Work out the finished part from the listing and answer in its coordinate system (mm). Face numbers are marked on the shaded views. Give positions to 0.01 mm unless a question says otherwise; leave off trailing zeros. Order: outer loops, then holes, each group sorted by start corner. A loop starts at its lowest first (then second) coordinate and runs counter-clockwise, first axis right, second up. Notation, with made-up numbers: (60, 75.25) -> (94, 75.25) arc R12 ccw to (94, 82.25) -> close; hole circle Ø2 at (21, 30). An arc over 180 degrees is marked (long way). Answer as CSV lines item,"result". Start each with the question number.
1. For a pull along X with two mould halves and no side action, classify the marked faces 1, 2 and 3 as released by +X, released by -X, zero draft, split by the parting line, or undercut.
2. A flat-ended cylindrical pin translates along its axis: pin 1 (2 mm diameter, centred on y = 13.5, z = 1.5, fed in from +X). Find the tip coordinate at first contact, or state that the pin passes through.
3. A cutting plane is placed at B-B (z = 2.5). State how many separate pieces and enclosed holes the cut face has, then the cut area to 3 significant figures.
4. A cutting plane is placed at A-A (x = -2). Give the vertices of the cut face in (y, z).
5. Find the intervals of material crossed by L1, parallel to X at y = -19, z = 4.5; L2, parallel to Y at x = -8, z = 2.2; L3, parallel to X at y = 24.5, z = 3.4, in increasing order.
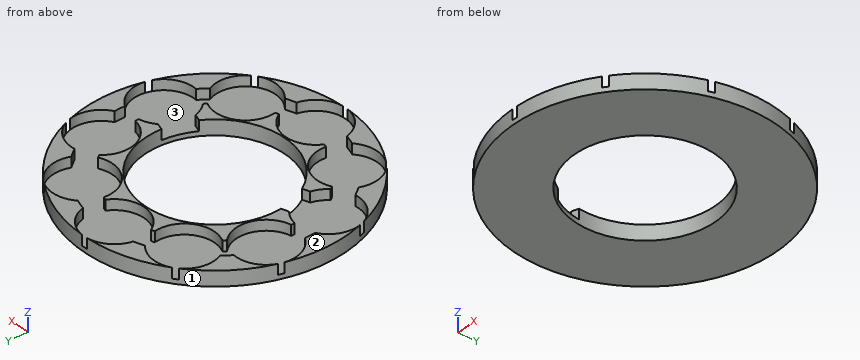
from build123d import *

# Parameters (mm, degrees)
SKETCH1_R                  = 42.14825
SKETCH1_R_2                = 22.5
BASIC_SHAPE_DEPTH          = 4.8
SKETCH2_R                  = 9.65
BATTERY_SLOT_DEPTH         = 3.3
BATTERY_SLOT_PATTERN_COUNT = 10
SKETCH3_R                  = 35.78
SKETCH3_R_2                = 29.28
BUS_SLOT_DEPTH             = 3.3
WIRE_SLIT_DEPTH            = 3.3


with BuildPart() as part:
    # Sketch1 → Basic Shape (new body)
    with BuildSketch(Plane.XY):
        Circle(SKETCH1_R)
        Circle(SKETCH1_R_2, mode=Mode.SUBTRACT)
    extrude(amount=BASIC_SHAPE_DEPTH)

    # Sketch2 → Battery Slot (cut)
    with BuildSketch(Plane.XY.offset(4.8)):
        with Locations((0, -32.53)):
            Circle(SKETCH2_R)
    battery_slot = extrude(amount=-BATTERY_SLOT_DEPTH, mode=Mode.SUBTRACT)

    # Battery Slot Pattern: Battery Slot ×10 about axis
    battery_slot_pattern_axis = Axis((0, 0, 0), (0, 0, 1))
    for i in range(1, BATTERY_SLOT_PATTERN_COUNT):
        add(battery_slot.rotate(battery_slot_pattern_axis, i * 360 / BATTERY_SLOT_PATTERN_COUNT), mode=Mode.SUBTRACT)

    # Sketch3 → Bus Slot (cut)
    with BuildSketch(Plane.XY.offset(4.8)):
        Circle(SKETCH3_R)
        Circle(SKETCH3_R_2, mode=Mode.SUBTRACT)
    extrude(amount=-BUS_SLOT_DEPTH, mode=Mode.SUBTRACT)

    # Sketch4 → Wire Slit (cut)
    with BuildSketch(Plane.XY.offset(4.8)):
        with BuildLine():
            Line((-24.633279562, -2.746526591), (-19.877996981, -1.201441619))
            Line((-19.877996981, -1.201441619), (-16.787827037, -10.712006782))
            Line((-16.787827037, -10.712006782), (-21.543109618, -12.257091754))
            ThreePointArc((-21.543109618, -12.257091754), (-21.760173093, -7.070308831), (-24.633279562, -2.746526591))
        make_face()
    wire_slit = extrude(amount=-WIRE_SLIT_DEPTH, mode=Mode.SUBTRACT)

    # Wire Slit Mirror: Wire Slit across plane
    add(wire_slit.mirror(Plane(origin=(0, 0, 0), x_dir=(0, 0, 1), z_dir=(1, 0, 0))), mode=Mode.SUBTRACT)


solid = part.part
Answer sheet:
1,face 1,"split by the parting line"
1,face 2,"zero draft"
1,face 3,"undercut"
2,pin 1,"stops at x = 40.25"
3,separate pieces,"12"
3,enclosed holes,"0"
3,area,"951 mm^2"
4,outline,"(-42.1, 0) -> (-22.41, 0) -> (-22.41, 4.8) -> (-23.09, 4.8) -> (-23.09, 1.5) -> (-41.97, 1.5) -> (-41.97, 4.8) -> (-42.1, 4.8) -> close; (22.41, 0) -> (42.1, 0) -> (42.1, 4.8) -> (41.97, 4.8) -> (41.97, 1.5) -> (23.09, 1.5) -> (23.09, 4.8) -> (22.41, 4.8) -> close"
5,L1,"x = -37.62 to -34.55, -12.83 to -12.05, 12.05 to 12.83, 34.55 to 37.62"
5,L2,"y = -41.38 to -37.93, -27.13 to -21.03, 21.03 to 27.13, 37.93 to 41.38"
5,L3,"x = -34.3 to -28.6, -9.64 to -5.35, 5.35 to 9.64, 28.6 to 34.3"
